Autodesk Inventor part; units mm, degrees
ref_plane "YZ Plane" through (0, 0, 0) normal (1, 0, 0) x (0, 1, 0)
ref_plane "XZ Plane" through (0, 0, 0) normal (0, 1, 0) x (-1, 0, 0)
ref_plane "XY Plane" through (0, 0, 0) normal (0, 0, 1) x (1, 0, 0)
sketch "Sketch1" plane through (0, 0, 0) normal (0, 0, 1) x (1, 0, 0)
  circle A0 centre (0, 0) radius 0.925
  line L0 (15, 2.6) -> (-0.8022, 3.4944)
  arc A1 (-0.8022, 3.4944) -> (-0.8022, -3.4944) centre (-1, 0) ccw
  line L1 (-0.8022, -3.4944) -> (15, -2.6)
  line L2 (0, 0) -> (26, 0) construction
  line L3 (15, 2.6) -> (66, 2.6)
  arc A2 (66, -2.6) -> (66, 2.6) centre (66, 0) ccw
  line L4 (66, -2.6) -> (15, -2.6)
  dimension "d0" = 1.85
  dimension "d7" = 3.5
  dimension "d8" = 1
  dimension "d10" = 2.6
  dimension "d11" = 66
  dimension "d12" = 16
extrude "Extrusion1" add sketch "Sketch1" along normal blind 3
properties part number "slider_link_p6"
Geometry: final body of the model. Coordinates: model frame, mm. A direction names the side the tool comes from. Round coordinates to 2 decimals unless told otherwise and drop trailing zeros. Loops run counter-clockwise (first coordinate to the right, second up) from the corner with the lowest first, then second, coordinate; pieces in that order, holes last.
Item 1: Mould query, pull axis X, two halves, no side actions, for faces 1 (the cylindrical face through (-0.201, 0.903, 1.479)), 2 (the flat face through (32, 0, 3)), 3 (the flat face through (7.21, 3.04, 1.48)). Classes: released by +X, released by -X, zero draft, split by the parting line, or undercut.
Checked values:
face 1: undercut
face 2: zero draft
face 3: released by +X
Item 2: Section D-D, the plane y = 1.75. Output: boundary loops of the cut face in (x, z).
Checked values:
outline: (-4.03, 0) - (67.92, 0) - (67.92, 3) - (-4.03, 3) - close
Item 3: Reachability of faces 4 (the flat face through (40, 2.6, 1)), 5 (the cylindrical face through (68.6, 0.1, 1.5)), 6 (the flat face through (41, -2.6, 1)) from +Z, -Z, +X, -X, +Y, -Y: full face, straight path, thin tool, end or side. Return the list, or none.
Checked values:
face 4: +Z, -Z, +X, +Y
face 5: +Z, -Z, +X
face 6: +Z, -Z, +X, -Y
Item 4: Line query: L1, parallel to Y at x = 45, z = 0.8; L2, parallel to X at y = 0.75, z = 2.7; L3, parallel to Y at x = 0, z = 1.05 (3 decimals). Output: solid intervals per line, ascending.
Checked values:
L1: y = -2.6 to 2.6
L2: x = -4.42 to -0.54, 0.54 to 68.49
L3: y = -3.449 to -0.925, 0.925 to 3.449
Item 5: Contact query for flat-ended pins moving along their axis: P1, Ø1.5, axis at x = 41, z = 2, coming from the -Y side; P2, Ø1.5, axis at x = 31, z = 1.5, coming from the +Y side; P3, Ø1.1, axis at x = 0, y = 0, coming from the -Z side. Output: stop coordinate, or through.
Checked values:
P1: stops at y = -2.6
P2: stops at y = 2.6
P3: passes through
Item 6: Section B-B, the plane x = 0. Output: boundary loops of the cut face in (y, z) (3 decimals), plus the area to 3 significant figures.
Checked values:
outline: (-3.449, 0) - (-0.925, 0) - (-0.925, 3) - (-3.449, 3) - close; (0.925, 0) - (3.449, 0) - (3.449, 3) - (0.925, 3) - close
area: 15.1 mm2
Item 7: Section C-C, the plane x = 41. Output: boundary loops of the cut face in (y, z).
Checked values:
outline: (-2.6, 0) - (2.6, 0) - (2.6, 3) - (-2.6, 3) - close
Item 8: Section A-A, the plane z = 0.95. Output: boundary loops of the cut face in (x, y) (3 decimals).
Checked values:
outline: (-0.802, -3.494) - (15, -2.6) - (66, -2.6) arc R2.6 ccw to (66, 2.6) - (15, 2.6) - (-0.802, 3.494) arc R3.5 ccw (long way) to start; hole circle Ø1.85 at (0, 0)
